Read the model definition and answer for the solid it produces. Units are mm, in the model's axes. A direction names the side the tool comes from. Coordinates: 2 decimals unless noted, no trailing zeros. Order: outer loops, then holes, each group sorted by start corner. A loop starts at its lowest first (then second) coordinate and runs counter-clockwise, first axis right, second up. Notation, with made-up numbers: (50, -3.75) - (105, -3.75) arc R24 ccw to (105, 18.25) - close; hole circle Ø3 at (-24, -30.5). An arc over 180 degrees is marked (long way). Write item = value, one per line.
from build123d import *

# Parameters (mm, degrees)
SKETCH1_R           = 20
BOSS_EXTRUDE1_DEPTH = 7.5
SKETCH2_R           = 20
SKETCH2_R_2         = 12.5
BOSS_EXTRUDE2_DEPTH = 15
SKETCH3_R           = 20
BOSS_EXTRUDE3_DEPTH = 10
CUT_EXTRUDE2_DEPTH  = 5
CUT_EXTRUDE3_DEPTH  = 44.084219849
SKETCH6_R           = 8
CUT_EXTRUDE4_DEPTH  = 5
SKETCH7_R           = 2.1
CUT_EXTRUDE5_DEPTH  = 4.5
SKETCH8_R           = 0.6
CUT_EXTRUDE6_DEPTH  = 41.868692174
FILLET1_R           = 1.5


with BuildPart() as part:
    # Sketch1 → Boss-Extrude1 (new body)
    with BuildSketch(Plane(origin=(0, 0, 0), x_dir=(1, 0, 0), z_dir=(0, 1, 0))):
        with Locations(Location((0, 0, 0), (0, 0, 270))):
            Circle(SKETCH1_R)
    extrude(amount=-BOSS_EXTRUDE1_DEPTH)

    # Sketch2 → Boss-Extrude2 (add)
    with BuildSketch(Plane.XZ.offset(7.5)):
        with Locations(Location((0, 0, 0), (0, 0, 90))):
            Circle(SKETCH2_R)
        with Locations(Location((0, 0, 0), (0, 0, 270))):
            Circle(SKETCH2_R_2, mode=Mode.SUBTRACT)
    extrude(amount=BOSS_EXTRUDE2_DEPTH)

    # Sketch3 → Boss-Extrude3 (add)
    with BuildSketch(Plane.XZ.offset(22.5)):
        with Locations(Location((0, 0, 0), (0, 0, 90))):
            Circle(SKETCH3_R)
    extrude(amount=BOSS_EXTRUDE3_DEPTH)

    # Sketch4 → Cut-Extrude2 (cut)
    with BuildSketch(Plane(origin=(0, -22.5, 0), x_dir=(-1, 0, 0), z_dir=(0, -1, 0))):
        Polygon((10.164510853, 5.47869076), (0.337570049, 11.542069996), (-9.826940805, 6.063379236), (-10.164510853, -5.47869076), (-0.337570049, -11.542069996), (9.826940805, -6.063379236), align=None)
    extrude(amount=CUT_EXTRUDE2_DEPTH, mode=Mode.SUBTRACT)

    # Sketch5 → Cut-Extrude3 (cut, through all)
    with BuildSketch(Plane(origin=(0, 0, 0), x_dir=(0, 0, -1), z_dir=(1, 0, 0))):
        Polygon((7.5, -17.5), (12.5, -17.5), (12.5, -7.5), (-12.5, -7.5), (-12.5, -17.5), (-7.5, -17.5), (-7.5, -32.5), (7.5, -32.5), align=None)
    extrude(amount=-CUT_EXTRUDE3_DEPTH, mode=Mode.SUBTRACT)

    # Sketch6 → Cut-Extrude4 (cut)
    with BuildSketch(Plane.XZ.offset(32.5)):
        Circle(SKETCH6_R)
    extrude(amount=-CUT_EXTRUDE4_DEPTH, mode=Mode.SUBTRACT)

    # Sketch7 → Cut-Extrude5 (cut)
    with BuildSketch(Plane.XZ.offset(7.5)):
        with Locations(Location((0, 0, 0), (0, 0, 270))):
            Circle(SKETCH7_R)
    extrude(amount=-CUT_EXTRUDE5_DEPTH, mode=Mode.SUBTRACT)

    # Sketch8 → Cut-Extrude6 (cut, through all)
    with BuildSketch(Plane.XZ.offset(3)):
        with Locations(Location((0, 0, 0), (0, 0, 270))):
            Circle(SKETCH8_R)
    extrude(amount=-CUT_EXTRUDE6_DEPTH, mode=Mode.SUBTRACT)

    # Fillet1
    fillet1_edges = [part.edges().sort_by_distance(p)[0] for p in [
        (0, -7.5, 2.1),
    ]]
    fillet(fillet1_edges, radius=FILLET1_R)


solid = part.part
1) Determine the mould class of faces 5 (the face through (0.631, -4.521, -2.003)), 6 (the face through (12.492, -16.562, -0.437)), 7 (the face through (0, -3, -1)) for opening direction Y: pulls with the +Y half, pulls with the -Y half, needs draft (parallel to the pull), parting line crosses it, or undercut.
Returned:
face_5 = needs draft
face_6 = undercut
face_7 = pulls with the -Y half
2) The part is cut by section A-A (z = 0). Determine the outline of the cut face in (x, y), and give its area (3 significant figures).
Returned:
outline = (-20, -7.5) - (-3.6, -7.5) arc R1.5 ccw to (-2.1, -6) - (-2.1, -3) - (-0.6, -3) - (-0.6, 0) - (-20, 0) - close; (0.6, -3) - (2.1, -3) - (2.1, -6) arc R1.5 ccw to (3.6, -7.5) - (12.5, -7.5) - (12.5, -22.5) - (10, -22.5) - (10, -27.5) - (8, -27.5) - (8, -32.5) - (20, -32.5) - (20, 0) - (0.6, 0) - close
area = 499 mm^2
3) For faces 1 (the face through (8, -30, 0)), 2 (the face through (-3.36, -24.96, 9.55)), 3 (the face through (-12, -27, 7.5)), 4 (the face through (-8, -12, 12.5)), determine the directions among +Z, -Z, +X, -X, +Y, -Y from which every point of the face is accessible in a straight line to the end or side of a thin tool.
Returned:
face_1 = -Y
face_2 = none
face_3 = -X, -Y
face_4 = -X
4) Straight lines are drawn through the part: line 1 along Z through (x, y) = (0, -11); line 2 along Z through (x, y) = (0, -30); line 3 along Y through (x, z) = (-9, -6). For each, find the intervals that lie inside material, in ascending order. Write a range as from..to.
Returned:
line_1 = -20..-12.5, 12.5..20
line_2 = -20..-8, 8..20
line_3 = -7.5..0
5) The part is cut by section B-B (y = -11.5). Determine the outline of the cut face in (x, z).
Returned:
outline = (-15.61, -12.5) arc R20 ccw (long way) to (-15.61, 12.5) - (0, 12.5) arc R12.5 cw to (0, -12.5) - close
6) The part is cut by section D-D (z = -10.5). Determine the outline of the cut face in (x, y), and give its area (3 significant figures).
Returned:
outline = (-17.02, -32.5) - (17.02, -32.5) - (17.02, 0) - (-17.02, 0) - (-17.02, -7.5) - (6.78, -7.5) - (6.78, -22.5) - (1.6, -22.5) - (1.6, -27.5) - (-2.03, -27.5) - (-2.03, -22.5) - (-6.78, -22.5) - (-6.78, -17.5) - (-17.02, -17.5) - close
area = 782 mm^2
7) Flat-ended cylindrical pins translate along their axes: pin 1 Ø1 at (y, z) = (-3.5, -10.5) entering from +X; pin 2 Ø4 at (y, z) = (-6, 1.5) entering from +X; pin 3 Ø1.1 at (x, z) = (0, 0) entering from +Y; pin 4 Ø7.5 at (x, y) = (-9.5, -21.5) entering from +Z. Find the tip coordinate at first contact, or state that the pin passes through.
Returned:
pin_1 = 17.32
pin_2 = 20
pin_3 = through
pin_4 = 19.16
8) The part is cut by section C-C (x = -4.5). Determine the outline of the cut face in (y, z), and give its area (3 significant figures).
Returned:
outline = (-32.5, -19.49) - (0, -19.49) - (0, 19.49) - (-32.5, 19.49) - (-32.5, 7.5) - (-27.5, 7.5) - (-27.5, 8.93) - (-22.5, 8.93) - (-22.5, 11.66) - (-17.5, 11.66) - (-17.5, 12.5) - (-7.5, 12.5) - (-7.5, -12.5) - (-17.5, -12.5) - (-17.5, -11.66) - (-22.5, -11.66) - (-22.5, -8.97) - (-27.5, -8.97) - (-27.5, -7.5) - (-32.5, -7.5) - close
area = 736 mm^2
